The drawing under review shows one solid part. Ordinate dimensions are in mm from its lowest x, y, z. A direction names the side the tool comes from. Coordinates: 2 decimals unless noted, no trailing zeros.
Q1. Insertion check: pin 1 (3 mm diameter, centred on x = 31.5, y = 15, fed in from +Z) (3 decimals); pin 2 (5.5 mm diameter, centred on x = 29.5, z = 12.5, fed in from +Y). Each pin has a flat end and moves straight along its axis. Give the tip position at first contact, or say it passes through.
Q2. Machinability: for the marked faces 1, 2 and 3, which of the approach directions +Z, -Z, +X, -X, +Y, -Y give a long, thin tool a straight path to every point of the face, cutting with its end or side? Answer none if there is none.
Q3. For probe 1 along Z at (x, y) = (7, 13) (1 decimal); probe 2 along Y at (x, z) = (30, 5) (1 decimal), list the stretches that pass through material, from the lowest coordinate up.
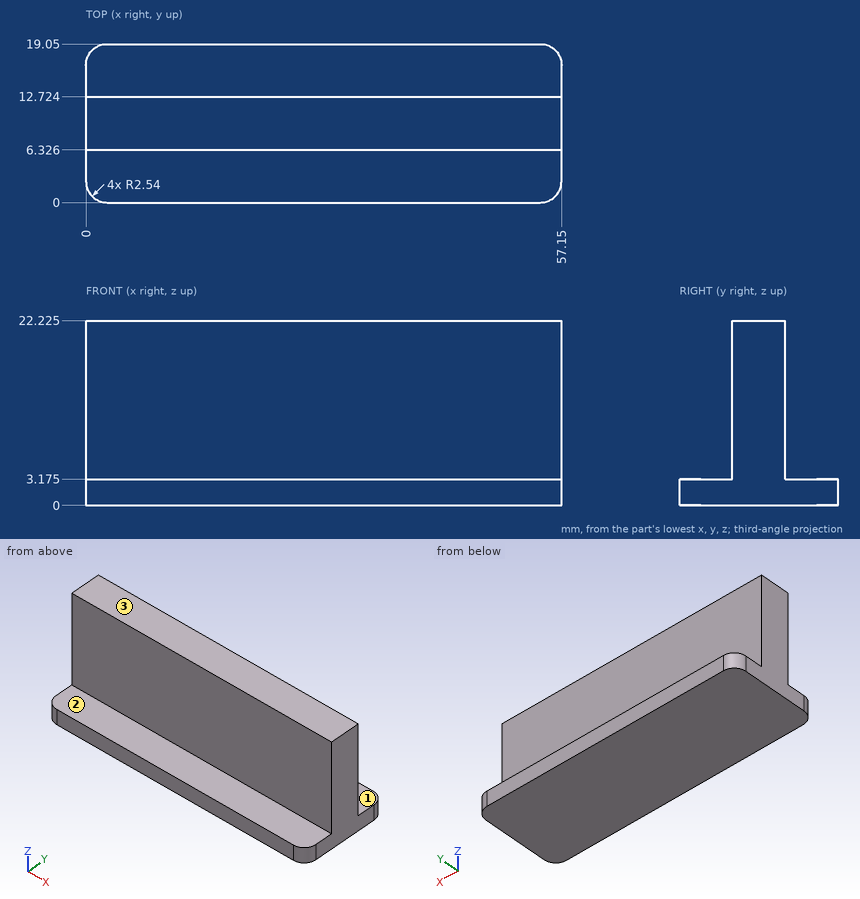
Response:
1. pin 1: stops at z = 3.175
1. pin 2: stops at y = 12.72
2. face 1: +Z, +X, -X, +Y
2. face 2: +Z, +X, -X, -Y
2. face 3: +Z, +X, -X, +Y, -Y
3. probe 1: z = 0 to 3.2
3. probe 2: y = 6.3 to 12.7
